from build123d import *

# Parameters (mm, degrees)
SKETCH_1_R      = 6.75
EXTRUDE_1_DEPTH = 10


with BuildPart() as part:
    # Эскиз1 → Бобышка-Вытянуть1 (new body)
    with BuildSketch(Plane.XY):
        with BuildLine():
            Line((469.898536303, 620), (469.898536303, 450))
            Line((469.898536303, 450), (484.898536303, 435))
            Line((484.898536303, 435), (589.898536303, 435))
            Line((589.898536303, 435), (604.898536303, 450))
            Line((604.898536303, 450), (604.898536303, 640))
            Line((604.898536303, 640), (589.898536303, 655))
            Line((589.898536303, 655), (569.898536303, 655))
            Line((569.898536303, 655), (552.827468491, 637.928932188))
            ThreePointArc((552.827468491, 637.928932188), (549.583235002, 635.761204675), (545.756400679, 635))
            Line((545.756400679, 635), (484.898536303, 635))
            Line((484.898536303, 635), (469.898536303, 620))
        make_face()
        with Locations((584.898536303, 455)):
            Circle(SKETCH_1_R, mode=Mode.SUBTRACT)
        with Locations((562.898536303, 455)):
            Circle(SKETCH_1_R, mode=Mode.SUBTRACT)
        with Locations((489.898536303, 455)):
            Circle(SKETCH_1_R, mode=Mode.SUBTRACT)
        with Locations((528.246102145, 476.749727554)):
            Circle(SKETCH_1_R, mode=Mode.SUBTRACT)
        with Locations((528.246102144, 528.249727554)):
            Circle(SKETCH_1_R, mode=Mode.SUBTRACT)
        with Locations((528.246102143, 575.749727554)):
            Circle(SKETCH_1_R, mode=Mode.SUBTRACT)
        with Locations((514.898536303, 615)):
            Circle(SKETCH_1_R, mode=Mode.SUBTRACT)
        with Locations((489.898536303, 615)):
            Circle(SKETCH_1_R, mode=Mode.SUBTRACT)
        with Locations((556.898536303, 615)):
            Circle(SKETCH_1_R, mode=Mode.SUBTRACT)
    extrude(amount=EXTRUDE_1_DEPTH)


solid = part.part
The model under review builds one solid part; all positions refer to its coordinate system, in mm. A direction names the side the tool comes from. Round coordinates to 2 decimals unless told otherwise and drop trailing zeros. Order: outer loops, then holes, each group sorted by start corner. A loop starts at its lowest first (then second) coordinate and runs counter-clockwise, first axis right, second up. Notation, with made-up numbers: (-20, 55.5) -> (-9, 55.5) arc R21 ccw to (-9, 82.5) -> close; hole circle Ø11 at (-35.5, -26.75). An arc over 180 degrees is marked (long way). Use CSV: the item, a comma, the result in double quotes. Start each with the question number.
(1) Consider section C-C on z = 8. State how many separate pieces and enclosed holes the cut face has, and give its area (3 significant figures).
(2) Consider section D-D on x = 580.5. Write out the cut boundary in (y, z).
(3) Tool access review of faces 1 (the face through (523, 580, 5)), 2 (the face through (516, 635, 5)): name each direction out of +Z, -Z, +X, -X, +Y, -Y from which nothing blocks a thin tool from reaching the whole face with its end or side.
(4) Consider section B-B on x = 517. Write out the cut boundary in (y, z), and give its area (3 significant figures).
(5) Consider section A-A on y = 455. Write out the cut boundary in (x, z).
(6) Mouldability with a two-part tool opening along Y and no side actions: class faces 3 (the face through (496.13, 452.41, 4.93)), 4 (the face through (597.5, 647.4, 4.9)), 5 (the face through (597.3, 442.4, 4.9)) as pulls with the +Y half, pulls with the -Y half, needs draft (parallel to the pull), parting line crosses it, or undercut.
(7) Insertion check: pin 1 (1.5 mm diameter, centred on x = 523, z = 5, fed in from +Y); pin 2 (21.5 mm diameter, centred on x = 556.9, y = 615, fed in from +Z). Each pin has a flat end and moves straight along its axis. Give the tip position at first contact, or say it passes through.
(8) Wall thickness on probe 1 along Y at (x, z) = (529, 6); probe 2 along X at (y, z) = (615, 5.5); probe 3 along X at (y, z) = (455, 5.5): over which ranges is each line inside the solid? List them lowest first. Write a range as from..to.
Responses:
1,separate pieces,"1"
1,enclosed holes,"9"
1,area,"26,200 mm²"
2,outline,"(435, 0) -> (449.88, 0) -> (449.88, 10) -> (435, 10) -> close; (460.12, 0) -> (655, 0) -> (655, 10) -> (460.12, 10) -> close"
3,face 1,"+Z, -Z"
3,face 2,"+Z, -Z, -X, +Y"
4,outline,"(435, 0) -> (608.59, 0) -> (608.59, 10) -> (435, 10) -> close; (621.41, 0) -> (635, 0) -> (635, 10) -> (621.41, 10) -> close"
4,area,"1,870 mm²"
5,outline,"(469.9, 0) -> (483.15, 0) -> (483.15, 10) -> (469.9, 10) -> close; (496.65, 0) -> (556.15, 0) -> (556.15, 10) -> (496.65, 10) -> close; (569.65, 0) -> (578.15, 0) -> (578.15, 10) -> (569.65, 10) -> close; (591.65, 0) -> (604.9, 0) -> (604.9, 10) -> (591.65, 10) -> close"
6,face 3,"undercut"
6,face 4,"pulls with the +Y half"
6,face 5,"pulls with the -Y half"
7,pin 1,"y = 635"
7,pin 2,"z = 10"
8,probe 1,"435..470.04, 483.46..521.54, 534.96..569.04, 582.46..635"
8,probe 2,"469.9..483.15, 496.65..508.15, 521.65..550.15, 563.65..604.9"
8,probe 3,"469.9..483.15, 496.65..556.15, 569.65..578.15, 591.65..604.9"
